Geometry: final body of the model. Coordinates: model frame, mm. A direction names the side the tool comes from. Round coordinates to 2 decimals unless told otherwise and drop trailing zeros. Loops run counter-clockwise (first coordinate to the right, second up) from the corner with the lowest first, then second, coordinate; pieces in that order, holes last. Notation, with made-up numbers: (-1.75, 68.25) - (33.25, 68.25) arc R21 ccw to (33.25, 101.25) - close; hole circle Ø7 at (20, 77.25). An arc over 180 degrees is marked (long way). Answer as a JSON object with one key per item and string values. Group by question number.
Item 1: Line query: line 1 (X direction, y = 1.25, z = -15); line 2 (X direction, y = 0.25, z = -16); line 3 (Y direction, x = 8, z = 20) (3 decimals). Output: solid intervals per line, ascending.
Item 2: Section B-B (z = -5.5). Return the cut outline in (x, y), plus the area to 3 significant figures.
Item 3: Section A-A (x = 2). Return the cut outline in (y, z) (1 decimal).
Item 4: First-contact query: pin 1 (1.3 mm diameter, centred on x = 11.5, y = 2, fed in from +Z); pin 2 (1.3 mm diameter, centred on y = -5.5, z = -15, fed in from +X); pin 3 (3 mm diameter, centred on x = -10, z = 0, fed in from +Y); pin 4 (4 mm diameter, centred on x = 27.68, z = 25.78, fed in from -Y). Flat tips, straight axial feed; report the tip coordinate or a pass-through.
Item 5: Reachability of faces 5 (the face through (12, 2, 21.969)), 6 (the face through (21.328, -5, -15)), 7 (the face through (28.948, 2, 13)), 8 (the face through (15, -5, -13.591)), 9 (the face through (12, 2, 4.189)) from +Z, -Z, +X, -X, +Y, -Y: full face, straight path, thin tool, end or side. Return the list, or none.
Item 6: Section C-C (y = -1). Return the cut outline in (x, z), plus the area to 3 significant figures.
Item 7: Section D-D (z = 23). Return the cut outline in (x, y).
Item 8: Draft query along Z for faces 1 (the face through (8.628, -5, -15)), 2 (the face through (29.13, 0.8, -5.16)), 3 (the face through (-24.645, 0.805, 25.712)), 4 (the face through (1, 1, 29.589)). Return one class per face: released by +Z, released by -Z, zero draft, split by the parting line, or undercut.
```python
from build123d import *

# Parameters (mm, degrees)
SKETCH1_W           = 60.96
SKETCH1_H           = 48.26
BOSS_EXTRUDE1_DEPTH = 1.5875
SKETCH2_W           = 33.02
SKETCH2_H           = 17.78
BOSS_EXTRUDE2_DEPTH = 1.5875
SKETCH3_R           = 1.524
CUT_EXTRUDE1_DEPTH  = 2.5875
SKETCH4_W           = 12.7
SKETCH4_H           = 2.54
BOSS_EXTRUDE3_DEPTH = 10.16


with BuildPart() as part:
    # Sketch1 → Boss-Extrude1 (new body)
    with BuildSketch(Plane(origin=(0, 0, 0), x_dir=(1, 0, 0), z_dir=(0, 1, 0))):
        with Locations((1.00761446, -5.459482072)):
            Rectangle(SKETCH1_W, SKETCH1_H)
    extrude(amount=BOSS_EXTRUDE1_DEPTH)

    # Sketch2 → Boss-Extrude2 (add)
    with BuildSketch(Plane(origin=(0, 1.5875, 0), x_dir=(1, 0, 0), z_dir=(0, 1, 0))):
        with Locations((12.43761446, -13.079482072)):
            Rectangle(SKETCH2_W, SKETCH2_H)
    extrude(amount=BOSS_EXTRUDE2_DEPTH)

    # Sketch3 → Cut-Extrude1 (cut, through all)
    with BuildSketch(Plane(origin=(0, 1.5875, 0), x_dir=(1, 0, 0), z_dir=(0, 1, 0))):
        with Locations((-23.12238554, 14.860517928)):
            Circle(SKETCH3_R)
        with Locations((27.67761446, 4.700517928)):
            Circle(SKETCH3_R)
        with Locations((-23.12238554, -25.779482072)):
            Circle(SKETCH3_R)
        with Locations((27.67761446, -25.779482072)):
            Circle(SKETCH3_R)
    extrude(amount=-CUT_EXTRUDE1_DEPTH, mode=Mode.SUBTRACT)

    # Sketch4 → Boss-Extrude3 (add)
    with BuildSketch(Plane(origin=(0, 0, 0), x_dir=(-1, 0, 0), z_dir=(0, -1, 0))):
        with Locations((-14.97761446, 14.860517928)):
            Rectangle(SKETCH4_W, SKETCH4_H)
    extrude(amount=BOSS_EXTRUDE3_DEPTH)


solid = part.part
```
Values:
{
 "1": {"line 1": "x = -29.47 to -24.64, -21.6 to 31.49", "line 2": "x = -29.47 to -24.13, -22.11 to 31.49", "line 3": "y = 0 to 3.175"},
 "2": {"outline": "(-29.47, 0) - (26.38, 0) - (26.38, 1.59) - (-29.47, 1.59) - close; (28.98, 0) - (31.49, 0) - (31.49, 1.59) - (28.98, 1.59) - close", "area": "92.7 mm^2"},
 "3": {"outline": "(0, -18.7) - (1.6, -18.7) - (1.6, 4.2) - (3.2, 4.2) - (3.2, 22) - (1.6, 22) - (1.6, 29.6) - (0, 29.6) - close"},
 "4": {"pin 1": "stops at z = 29.59", "pin 2": "stops at x = 21.33", "pin 3": "stops at y = 1.59", "pin 4": "stops at y = 0"},
 "5": {"face 5": "+Z, +X, -X, +Y", "face 6": "+Z, -Z, +X, -Y", "face 7": "+Z, -Z, +X, +Y", "face 8": "+Z, +X, -X, -Y", "face 9": "-Z, +X, -X, +Y"},
 "6": {"outline": "(8.63, -16.13) - (21.33, -16.13) - (21.33, -13.59) - (8.63, -13.59) - close", "area": "32.3 mm^2"},
 "7": {"outline": "(-29.47, 0) - (31.49, 0) - (31.49, 1.59) - (-29.47, 1.59) - close"},
 "8": {"face 1": "zero draft", "face 2": "undercut", "face 3": "undercut", "face 4": "released by +Z"}
}
